Part model, mm, in its own coordinate system. A direction names the side the tool comes from. Coordinates: 2 decimals unless noted, no trailing zeros. Order: outer loops, then holes, each group sorted by start corner. A loop starts at its lowest first (then second) coordinate and runs counter-clockwise, first axis right, second up. Notation, with made-up numbers: M -14,38.5 L 11,38.5 A19 ccw 11,49.5 Z; hole C 37,60 d10. An arc over 180 degrees is marked long. Answer in a Markdown table with one row per item. Add a question column.
from build123d import *

# Parameters (mm, degrees)
F1_DEPTH = 38.1
F2_DEPTH = 63.5
F3_R     = 5.08
F4_W     = 89.9337530136
F4_H     = 74.9955805898
F5_DEPTH = 25.4
F6_R     = 5.08


with BuildPart() as f1:
    # F0 (on Top) → F1 (new body)
    with BuildSketch(Plane.XY):
        with BuildLine():
            Line((67.3384442925, 44.9668765068), (-67.3384442925, 44.9668765068))
            Line((-67.3384442925, 44.9668765068), (-67.3384442925, 44.7683221654))
            ThreePointArc((-67.3384442925, 44.7683221654), (-35.682460107, 31.6559841855), (-22.5701221271, 0))
            ThreePointArc((-22.5701221271, 0), (-35.682460107, -31.6559841855), (-67.3384442925, -44.7683221654))
            Line((-67.3384442925, -44.7683221654), (-67.3384442925, -44.9668765068))
            Line((-67.3384442925, -44.9668765068), (67.3384442925, -44.9668765068))
            Line((67.3384442925, -44.9668765068), (67.3384442925, 44.9668765068))
        make_face()
    extrude(amount=F1_DEPTH)

    # F0 (on Top) → F2 (join)
    with BuildSketch(Plane.XY):
        with BuildLine():
            Line((-67.3384442925, 21.3704215864), (-67.3384442925, 44.7683221654))
            ThreePointArc((-67.3384442925, 44.7683221654), (-112.1067664579, 0), (-67.3384442925, -44.7683221654))
            Line((-67.3384442925, -44.7683221654), (-67.3384442925, -21.3704215864))
            ThreePointArc((-67.3384442925, -21.3704215864), (-88.7088658789, 0), (-67.3384442925, 21.3704215864))
        make_face()
        with BuildLine():
            ThreePointArc((-22.5701221271, 0), (-35.682460107, 31.6559841855), (-67.3384442925, 44.7683221654))
            Line((-67.3384442925, 44.7683221654), (-67.3384442925, 21.3704215864))
            ThreePointArc((-67.3384442925, 21.3704215864), (-52.227274272, 15.1111700206), (-45.9680227061, 0))
            ThreePointArc((-45.9680227061, 0), (-52.227274272, -15.1111700206), (-67.3384442925, -21.3704215864))
            Line((-67.3384442925, -21.3704215864), (-67.3384442925, -44.7683221654))
            ThreePointArc((-67.3384442925, -44.7683221654), (-35.682460107, -31.6559841855), (-22.5701221271, 0))
        make_face()
    extrude(amount=F2_DEPTH)

    # F3
    f3_edges = [f1.edges().sort_by_distance(p)[0] for p in [
        (-67.338444, 44.768322, 63.5),
    ]]
    fillet(f3_edges, radius=F3_R)

    # F4 (on face) → F5 (join)
    with BuildSketch(Plane.YZ.offset(67.3384442925)):
        with Locations((0, 0.6022097051)):
            Rectangle(F4_W, F4_H)
    extrude(amount=F5_DEPTH)

    # F6
    f6_edges = [f1.edges().sort_by_distance(p)[0] for p in [
        (92.738444, -44.966877, 0.60221),
        (67.338444, -44.966877, -18.44779),
        (92.738444, 0, -36.895581),
    ]]
    fillet(f6_edges, radius=F6_R)


solid = f1.part
(1) Slice it at D-D (z = 48). List the corners of the cut face in (x, y).
(2) 3-axis set-ups, long thin cutter, end or side, ignore diameter. For faces 1 (the cylindrical face through (68.87, -43.52, -18.19)), 2 (the cylindrical face through (-111.042, 9.705, 35.292)), 3 (the flat face through (67.338, 2, -18)): which of +Z, -Z, +X, -X, +Y, -Y reach the whole face in a straight line?
(3) Slice it at A-A (z = 30). List the corners of the cut face in (x, y).
(4) Slice it at C-C (x = 55). List the corners of the cut face in (y, z).
(5) Wall check: line 1 (Z direction, x = -91, y = 20.5); line 2 (Z direction, x = -11.5, y = -32); line 3 (Y direction, x = -71.5, z = 28). Give the ranges that are in metal, low to high.
(6) Slice it at B-B (z = -29.5). List the corners of the cut face in (x, y).
(7) Drop flat-ended pins along their axis: P1, Ø6, axis at y = -31, z = 40.5, coming from the -X side; P2, Ø6, axis at x = 16, y = 0, coming from the -Z side; P3, Ø18.5, axis at y = 16, z = -16.5, coming from the -X side. Give the stop position or say it passes through.
Computed:
| question | item | result |
|---|---|---|
| 1 | outline | C -67.34,0 d89.54; hole C -67.34,0 d42.74 |
| 2 | face 1 | -Z, -X, -Y |
| 2 | face 2 | +Z |
| 2 | face 3 | -Z, -X, +Y, -Y |
| 3 | outline | M -67.34,-44.97 L 87.66,-44.97 A5.08 ccw 92.74,-39.89 L 92.74,44.97 L -67.34,44.97 L -67.34,44.77 A44.77 ccw -67.34,-44.77 Z; hole C -67.34,0 d42.74 |
| 4 | outline | M -44.97,0 L 44.97,0 L 44.97,38.1 L -44.97,38.1 Z |
| 5 | line 1 | z = 0 to 63.5 |
| 5 | line 2 | z = 0 to 38.1 |
| 5 | line 3 | y = -44.57 to -20.96, 20.96 to 44.57 |
| 6 | outline | M 67.34,-39.89 A5.08 ccw 72.42,-44.97 L 87.66,-44.97 A5.08 ccw 92.74,-39.89 L 92.74,44.97 L 67.34,44.97 Z |
| 7 | P1 | stops at x = -102.27 |
| 7 | P2 | stops at z = 0 |
| 7 | P3 | stops at x = 67.34 |
